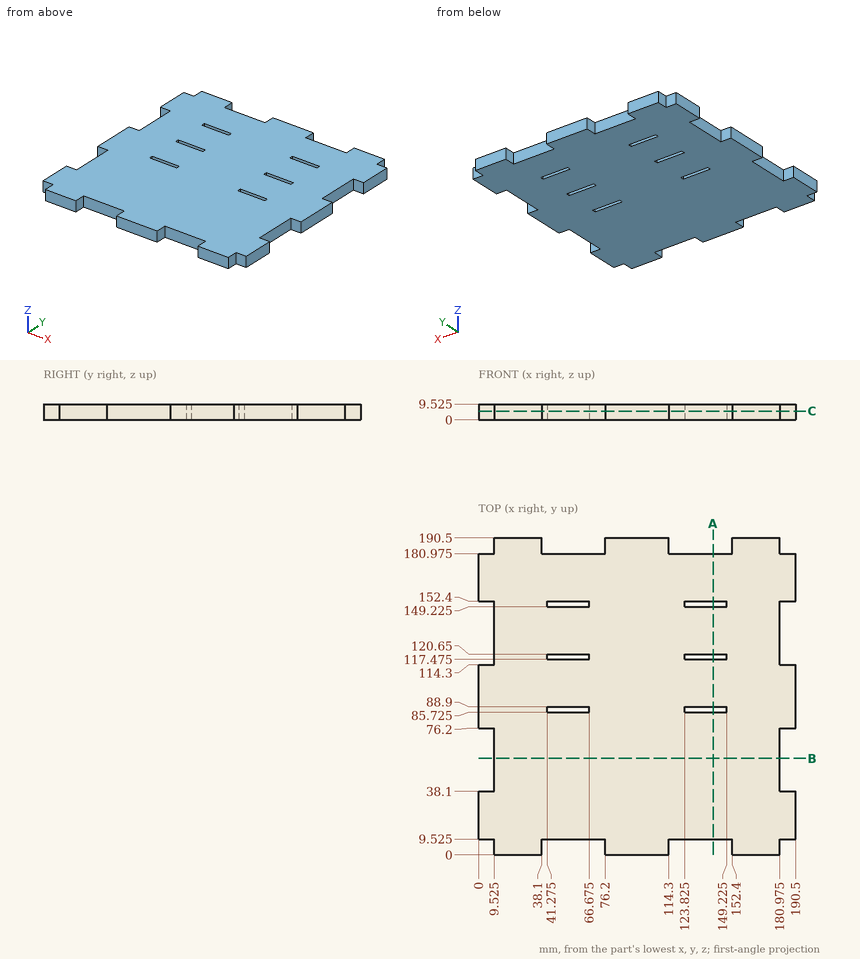
Part print with two shaded views. Sizes in mm from the minimum x, y, z corner. Round coordinates to 2 decimals unless told otherwise and drop trailing zeros. Loops run counter-clockwise (first coordinate to the right, second up) from the corner with the lowest first, then second, coordinate; pieces in that order, holes last.
Item 1: Drill centre lines: line 1 along Y through (x, z) = (53.5, 1.75) (3 decimals); line 2 along Y through (x, z) = (120.5, 8.5) (3 decimals). Where is each one in solid material? Low to high.
Item 2: Saw through at C-C (z = 5.25). State how many separate pieces and enclosed holes the cut face has, then the cut area to 3 significant figures.
Item 3: Pin check, flat tips, straight feed: P1, Ø5, axis at y = 70, z = 3.5, coming from the -X side (3 decimals); P2, Ø5, axis at x = 138, z = 3, coming from the +Y side (3 decimals); P3, Ø3, axis at x = 131, z = 6.5, coming from the -Y side (3 decimals). Stop position of each tip, or through.
Item 4: Saw through at B-B (y = 58). List the corners of the cut face in (x, z) (3 decimals), then the cut area to 3 significant figures.
Item 5: Saw through at A-A (x = 141). List the corners of the cut face in (y, z) (3 decimals).
Worked answers:
1. line 1: y = 9.525 to 85.725, 88.9 to 117.475, 120.65 to 149.225, 152.4 to 180.975
1. line 2: y = 9.525 to 180.975
2. separate pieces: 1
2. enclosed holes: 6
2. area: 32,500 mm2
3. P1: stops at x = 9.525
3. P2: stops at y = 180.975
3. P3: stops at y = 9.525
4. outline: (9.525, 0) - (180.975, 0) - (180.975, 9.525) - (9.525, 9.525) - close
4. area: 1,630 mm2
5. outline: (9.525, 0) - (85.725, 0) - (85.725, 9.525) - (9.525, 9.525) - close; (88.9, 0) - (117.475, 0) - (117.475, 9.525) - (88.9, 9.525) - close; (120.65, 0) - (149.225, 0) - (149.225, 9.525) - (120.65, 9.525) - close; (152.4, 0) - (180.975, 0) - (180.975, 9.525) - (152.4, 9.525) - close
